Source: CAD feature listing. Evaluate the final solid. Frame: model axes, mm. Coordinates: 2 decimals unless noted, no trailing zeros. Write each loop counter-clockwise with the first axis right and the second up, starting at its lowest first coordinate (ties: lowest second). Pieces come first, ordered by that corner, then holes. Notation, with made-up numbers: M 58.5,-39.75 L 102.5,-39.75 A15 ccw 102.5,-25.75 Z; hole C 30,23 d7. An arc over 180 degrees is marked long. Answer as CSV lines item,"result". Start each with the question number.
1. Line query: probe 1 along X at (y, z) = (-3.75, 115); probe 2 along Z at (x, y) = (150.5, -3.25); probe 3 along Z at (x, y) = (-150.5, -3.45). Output: solid intervals per line, ascending. Write a range as [from, to].
2. Section A-A on z = 69. Return the cut outline in (x, y).
3. Section C-C on x = -103. Return the cut outline in (y, z), plus the area to 3 significant figures.
4. Section B-B on y = -2.15. Return the cut outline in (x, z).
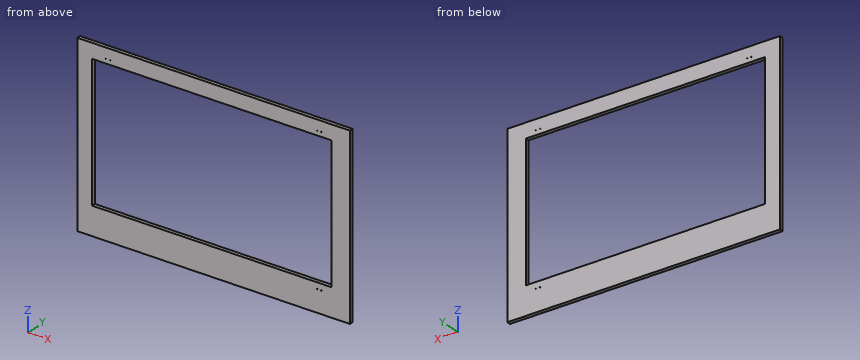
```python
from build123d import *

# Parameters (mm, degrees)
F0_W     = 396
F0_H     = 260
F0_R     = 0.5
F0_W_2   = 347.75
F0_H_2   = 197.5
F1_DEPTH = 5.5


with BuildPart() as f1:
    # F0 (on Front) → F1 (new body)
    with BuildSketch(Plane.XZ):
        Rectangle(F0_W, F0_H)
        with Locations((150.5, -98)):
            Circle(F0_R, mode=Mode.SUBTRACT)
        with Locations((156.5, -98)):
            Circle(F0_R, mode=Mode.SUBTRACT)
        with Locations((-2.625, 9.75)):
            Rectangle(F0_W_2, F0_H_2, mode=Mode.SUBTRACT)
        with Locations((-156.5, 115)):
            Circle(F0_R, mode=Mode.SUBTRACT)
        with Locations((-150.5, 115)):
            Circle(F0_R, mode=Mode.SUBTRACT)
        with Locations((150.5, 115)):
            Circle(F0_R, mode=Mode.SUBTRACT)
        with Locations((156.5, 115)):
            Circle(F0_R, mode=Mode.SUBTRACT)
    extrude(amount=F1_DEPTH)


solid = f1.part
```
Values:
1,probe 1,"[-198, -157], [-156, -151], [-150, 150], [151, 156], [157, 198]"
1,probe 2,"[-130, -98.5], [-97.5, -89], [108.5, 114.5], [115.5, 130]"
1,probe 3,"[-130, -89], [108.5, 114.5], [115.5, 130]"
2,outline,"M -198,-5.5 L -176.5,-5.5 L -176.5,0 L -198,0 Z; M 171.25,-5.5 L 198,-5.5 L 198,0 L 171.25,0 Z"
3,outline,"M -5.5,-130 L 0,-130 L 0,-89 L -5.5,-89 Z; M -5.5,108.5 L 0,108.5 L 0,130 L -5.5,130 Z"
3,area,"344 mm²"
4,outline,"M -198,-130 L 198,-130 L 198,130 L -198,130 Z; hole M -176.5,-89 L 171.25,-89 L 171.25,108.5 L -176.5,108.5 Z; hole C -156.5,115 d1; hole C -150.5,115 d1; hole C 150.5,-98 d1; hole C 150.5,115 d1; hole C 156.5,-98 d1; hole C 156.5,115 d1"
